The listing builds one solid part. Answer for the finished solid, in the listing's coordinates (mm). Face numbers are marked on the shaded views. Coordinates: 2 decimals unless noted, no trailing zeros. Order: outer loops, then holes, each group sorted by start corner. A loop starts at its lowest first (then second) coordinate and runs counter-clockwise, first axis right, second up. Notation, with made-up numbers: (34.25, 62) -> (42.25, 62) arc R13 ccw to (42.25, 72) -> close; hole circle Ø4 at (61, -32.5). An arc over 180 degrees is marked (long way). Put each result on its own line as item: value. Start each with the question number.
Autodesk Inventor part; units mm, degrees
ref_plane "YZ Plane" through (0, 0, 0) normal (1, 0, 0) x (0, 1, 0)
ref_plane "XY Plane" through (0, 0, 0) normal (0, 0, 1) x (1, 0, 0)
sketch "Sketch1" plane through (0, 0, 0) normal (0, 0, 1) x (1, 0, 0)
  arc A0 (32.6355, 29.9298) -> (29.3759, 33.1607) centre (29.5384, 30.0649) ccw
  arc A1 (27.8274, -32.2191) -> (30.1546, -26.93) centre (30.0194, -30.0271) ccw
  arc A2 (32.4933, 26.671) -> (34.0351, 30.2371) centre (29.5384, 30.0649) ccw
  arc A3 (26.8375, -33.2091) -> (34.5127, -29.7804) centre (30.0194, -30.0271) ccw
  line L0 (-29.9673, 30.0452) -> (-33.1472, 26.8653)
  line L1 (-29.9673, 30.0452) -> (-25.4702, 30.0452) construction
  line L2 (-29.9673, 30.0452) -> (-21.8579, 30.471)
  line L3 (30.0194, -30.0271) -> (30.3698, -21.9984)
  line L4 (30.0194, -30.0271) -> (26.8375, -33.2091)
  circle A4 centre (0, 0) radius 37.5
  arc A5 (34.5127, -29.7804) -> (34.0351, 30.2371) centre (-61.1139, -0.5306) ccw
  arc A6 (29.3158, 34.5594) -> (-29.9754, 34.5423) centre (-0.3022, -60.9538) ccw
  line L5 (18.5473, 32.5922) -> (29.3759, 33.1607)
  line L6 (32.1704, 19.2696) -> (32.6355, 29.9298)
  arc A7 (29.3158, 34.5594) -> (26.1185, 32.9896) centre (29.5384, 30.0649) ccw
  arc A8 (34.0351, 30.2371) -> (29.3158, 34.5594) centre (29.5384, 30.0649) ccw
  arc A9 (-29.9754, 34.5423) -> (-33.1472, 26.8653) centre (-29.9673, 30.0452) ccw
  arc A10 (-26.8454, 30.2091) -> (-32.1778, 27.8347) centre (-29.9673, 30.0452) ccw
  dimension "d0" = 6.2
  dimension "d1" = 6.2
  dimension "d6" = 9
  dimension "d7" = 9
  dimension "d8" = 135
  dimension "d9" = 75
  dimension "d11" = 100
  dimension "d12" = 100
extrude "Extrusion1" add sketch "Sketch1" along normal blind 100 contours A0 L5 A7 A8 A2 L6 | A2 A5 A3 L4 A1 L3 A4 L6 | L5 A4 L2 A10 L0 A9 A6 A7
ref_plane "Work Plane1" through (0, 27, 0) normal (0, 1, 0) x (-1, 0, 0)
split "Split1" plane through (0, 27, 0) removes the side toward (0, -1, 0)
properties part number "Cage60mm-2sides-InnerD75mm-L100mm"
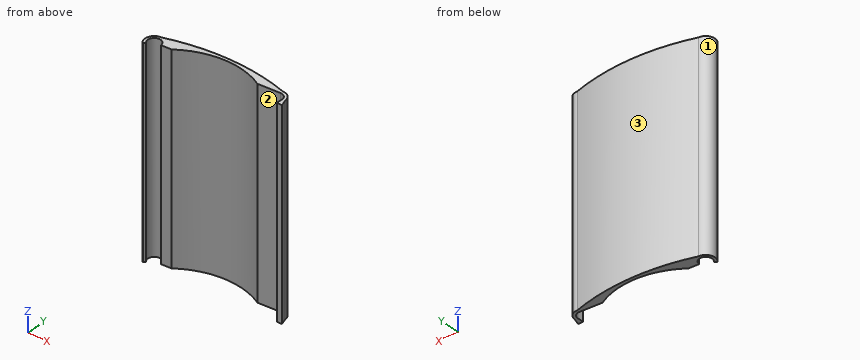
(1) The part is cut by section B-B on z = 65. Determine the outline of the cut face in (x, y).
(2) The part is cut by section D-D on x = -5.5. Determine the outline of the cut face in (y, z).
(3) Each of these flat-tipped pins is pushed along its axis until it touches: P1, Ø5, axis at y = 33.5, z = 10.5, coming from the -X side; P2, Ø5, axis at y = 34.5, z = 19, coming from the +X side; P3, Ø8, axis at x = 18, z = 80, coming from the -Y side. Where does it stop, or does it pass through?
(4) The part is cut by section C-C on x = 21. Determine the outline of the cut face in (y, z).
(5) Find the intervals of material crossed by L1, parallel to X at y = 31.5, z = 23; L2, parallel to X at y = 30.5, z = 69; L3, parallel to X at y = 33.5, z = 94.5, in increasing order.
(6) For a pull along X with two mould halves and no side action, classify the marked faces 1, 2 and 3 as released by +X, released by -X, zero draft, split by the parting line, or undercut.
(7) The part is cut by section A-A on y = 35.75. Determine the outline of the cut face in (x, z).
Worked out:
1. outline: (-33.28, 27) -> (-33.01, 27) -> (-32.18, 27.83) arc R3.13 cw (long way) to (-26.85, 30.21) -> (-21.86, 30.47) arc R37.5 cw to (18.55, 32.59) -> (29.38, 33.16) arc R3.1 cw to (32.64, 29.93) -> (32.51, 27) -> (35.02, 27) arc R100 ccw to (34.04, 30.24) arc R4.5 ccw to (29.32, 34.56) arc R100 ccw to (-29.98, 34.54) arc R4.5 ccw to start
2. outline: (37.09, 0) -> (38.91, 0) -> (38.91, 100) -> (37.09, 100) -> close
3. P1: x = -34.36
3. P2: x = 33.6
3. P3: y = 32.59
4. outline: (32.72, 0) -> (36.75, 0) -> (36.75, 100) -> (32.72, 100) -> close
5. L1: -34.22 to -32.73, -27.2 to -20.35, 32.29 to 33.8
5. L2: -34.44 to -33.06, -26.87 to -21.82, 32.61 to 34.02
5. L3: -32.85 to -16.85, 16.85 to 32.45
6. face 1: released by -X
6. face 2: undercut
6. face 3: split by the parting line
7. outline: (-25.77, 0) -> (-11.32, 0) -> (-11.32, 100) -> (-25.77, 100) -> close; (11.32, 0) -> (25.16, 0) -> (25.16, 100) -> (11.32, 100) -> close
